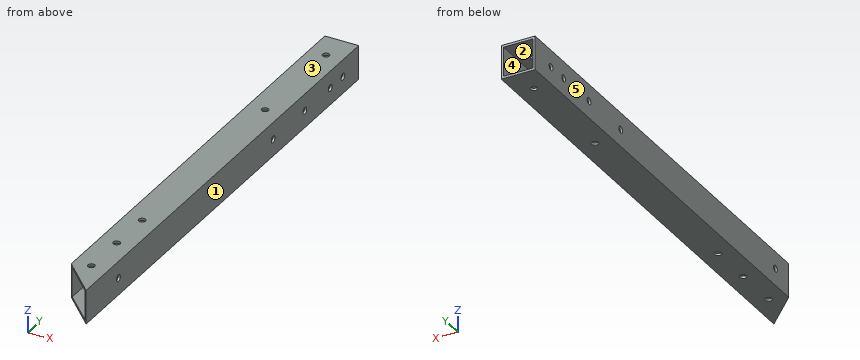
from build123d import *

# Parameters (mm, degrees)
SKETCH_1_W          = 15
SKETCH_1_H          = 15
SKETCH_1_W_2        = 13
SKETCH_1_H_2        = 13
EXTRUDE_1_DEPTH     = 215
SKETCH_2_R          = 1.5
CUT_EXTRUDE_1_DEPTH = 216.653077882
SKETCH_3_R          = 1.5
CUT_EXTRUDE_2_DEPTH = 216.653077882


with BuildPart() as part:
    # 草图1 → 凸台-拉伸1 (new body)
    with BuildSketch(Plane(origin=(0, 0, 0), x_dir=(1, 0, 0), z_dir=(0, 1, 0))):
        Rectangle(SKETCH_1_W, SKETCH_1_H)
        Rectangle(SKETCH_1_W_2, SKETCH_1_H_2, mode=Mode.SUBTRACT)
    extrude(amount=EXTRUDE_1_DEPTH)

    # 草图2 → 切除-拉伸1 (cut, through all)
    with BuildSketch(Plane.XY.offset(7.5)):
        with Locations((0, 37.5)):
            Circle(SKETCH_2_R)
        with Locations((0, 17.5)):
            Circle(SKETCH_2_R)
        with Locations((0, 57.5)):
            Circle(SKETCH_2_R)
        with Locations((0, 202.5)):
            Circle(SKETCH_2_R)
        with Locations((0, 154.5)):
            Circle(SKETCH_2_R)
        Polygon((7.5, 0), (-7.5, 0), (-7.5, 15), align=None)
    extrude(amount=-CUT_EXTRUDE_1_DEPTH, mode=Mode.SUBTRACT)

    # 草图3 → 切除-拉伸2 (cut, through all)
    with BuildSketch(Plane(origin=(7.5, 0, 0), x_dir=(0, 0, -1), z_dir=(1, 0, 0))):
        with Locations((0, 172.5)):
            Circle(SKETCH_3_R)
        with Locations((0, 192.5)):
            Circle(SKETCH_3_R)
        with Locations((0, 147.5)):
            Circle(SKETCH_3_R)
        with Locations((0, 202.5)):
            Circle(SKETCH_3_R)
        with Locations((0, 25.5)):
            Circle(SKETCH_3_R)
    extrude(amount=-CUT_EXTRUDE_2_DEPTH, mode=Mode.SUBTRACT)


solid = part.part
Model file for the job. Use its own axes, mm. Face numbers are marked on the shaded views. A direction names the side the tool comes from. Give positions to 0.01 mm unless a question says otherwise; leave off trailing zeros. Write each loop counter-clockwise with the first axis right and the second up, starting at its lowest first coordinate (ties: lowest second). Pieces come first, ordered by that corner, then holes. Notation, with made-up numbers: (86.25, 67.5) - (122.25, 67.5) arc R35 ccw to (122.25, 99.5) - close; hole circle Ø5 at (60.25, -5). An arc over 180 degrees is marked (long way). Answer as CSV lines item,"result".
1. Pin check, flat tips, straight feed: pin 1 (1.8 mm diameter, centred on y = 25.5, z = 0, fed in from -X); pin 2 (6 mm diameter, centred on x = -3, z = 5, fed in from -Y); pin 3 (8 mm diameter, centred on x = 0, z = -5, fed in from -Y). Stop position of each tip, or through.
Responses:
pin 1,"passes through"
pin 2,"stops at y = 7.9"
pin 3,"stops at y = 3.79"
2. Two-plate mould, pull along Z, no slides. Class the marked faces 3, 4 and 5: +Z half, -Z half, draft (parallel to the pull), parting line (faces both ways), or undercut.
Responses:
face 3,"+Z half"
face 4,"undercut"
face 5,"draft"
3. Band-saw the part on B-B (y = 53.5). Write the cut outline in (x, z).
Responses:
outline,"(-7.5, -7.5) - (7.5, -7.5) - (7.5, 7.5) - (-7.5, 7.5) - close; hole (-6.5, -6.5) - (6.5, -6.5) - (6.5, 6.5) - (-6.5, 6.5) - close"
4. 3-axis set-ups, long thin cutter, end or side, ignore diameter. For the marked faces 1 and 2: which of +Z, -Z, +X, -X, +Y, -Y reach the whole face in a straight line?
Responses:
face 1,"+Z, -Z, +X, +Y, -Y"
face 2,"+Y, -Y"
5. Band-saw the part on A-A (x = 4.75). Write the cut outline in (y, z), and give its area (4 significant figures).
Responses:
outline,"(2.75, -7.5) - (215, -7.5) - (215, -6.5) - (2.75, -6.5) - close; (2.75, 6.5) - (215, 6.5) - (215, 7.5) - (2.75, 7.5) - close"
area,"424.5 mm2"
6. Drill centre lines: L1, parallel to Y at x = 0, z = -6.8; L2, parallel to X at y = 202.5, z = -6.65; L3, parallel to Y at x = -7.1, z = 0. Where is each one in solid material? Low to high. Write a range as [from, to].
Responses:
L1,"y = [7.5, 16], [19, 36], [39, 56], [59, 153], [156, 201], [204, 215]"
L2,"x = [-7.5, -1.5], [1.5, 7.5]"
L3,"y = [14.6, 24], [27, 146], [149, 171], [174, 191], [194, 201], [204, 215]"
